Input: dimensioned drawing with shaded views. Units: mm. Origin: part minimum x, y, z. A direction names the side the tool comes from. Coordinates: 2 decimals unless noted, no trailing zeros. Loops run counter-clockwise (first coordinate to the right, second up) from the corner with the lowest first, then second, coordinate; pieces in that order, holes last. Notation, with made-up numbers: (-29.75, 77.5) - (-4.75, 77.5) arc R12 cw to (-4.75, 92.5) - close; hole circle Ø5 at (32, -16.5). An arc over 180 degrees is marked (long way). Put each result on its own line as item: value. Start each with the question number.
1) Contact query for flat-ended pins moving along their axis: pin 1 Ø1 at (x, z) = (4, 11) entering from +Y (1 decimal); pin 2 Ø3 at (x, z) = (2, 16) entering from +Y; pin 3 Ø3 at (y, z) = (11, 13.5) entering from -X. Output: stop coordinate, or through.
2) Reachability of the marked faces 4 and 5 from +Z, -Z, +X, -X, +Y, -Y: full face, straight path, thin tool, end or side. Return the list, or none.
3) Section A-A on y = 3.5. Output: boundary loops of the cut face in (x, z).
4) Section D-D on y = 16. Output: boundary loops of the cut face in (x, z).
5) Material intervals for line 1 along Y through (x, z) = (4.4, 4); line 2 along Z through (x, y) = (3.2, 12); line 3 along Z through (x, y) = (4.55, 20.5), sorted ascending. Write a range as from..to.
6) Section C-C on x = 3.8. Output: boundary loops of the cut face in (y, z), and give its area (3 significant figures).
7) Section B-B on z = 4. Output: boundary loops of the cut face in (x, y).
8) Draft query along Z for the marked faces 1, 2 and 3. Return one class per face: +Z half, -Z half, draft (parallel to the pull), parting line (faces both ways), or undercut.
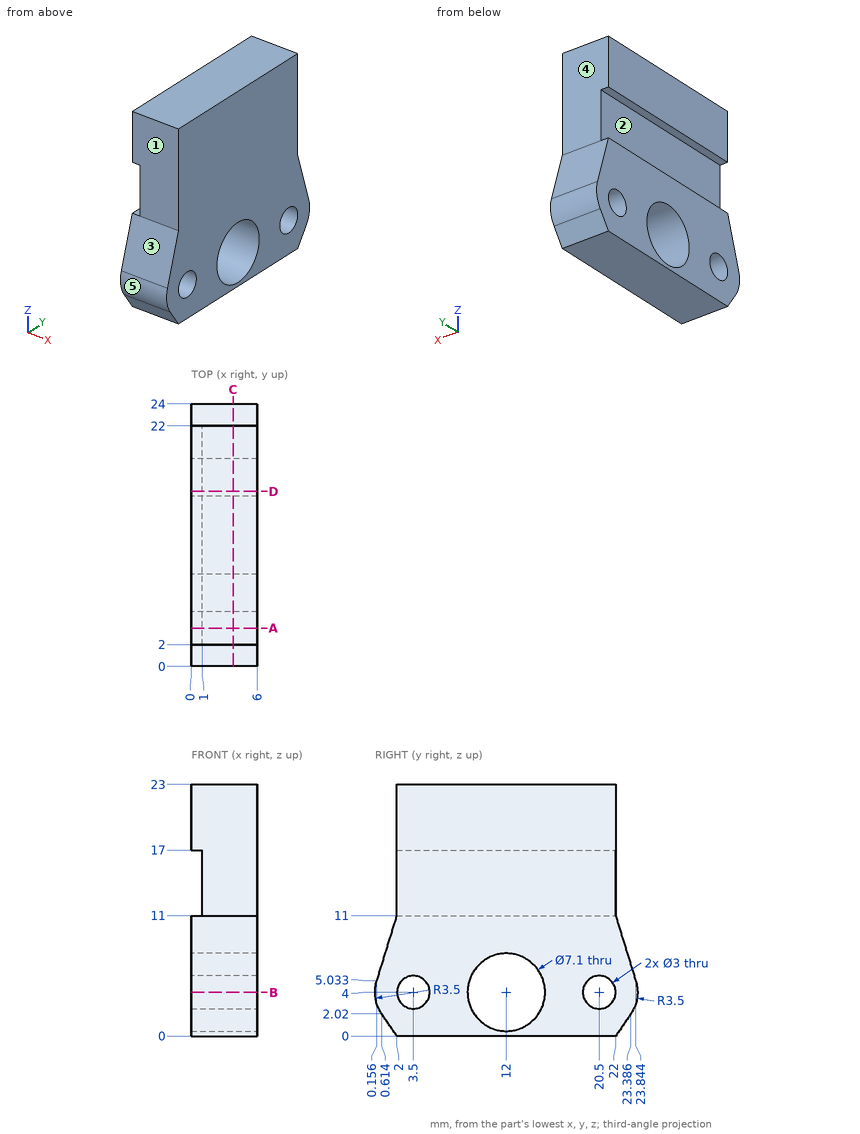
Answer block:
1. pin 1: stops at y = 22.2
1. pin 2: stops at y = 22
1. pin 3: stops at x = 1
2. face 4: +Z, +X, -X, +Y
2. face 5: +X, -X, -Y
3. outline: (0, 0) - (6, 0) - (6, 2.5) - (0, 2.5) - close; (0, 5.5) - (6, 5.5) - (6, 23) - (0, 23) - (0, 17) - (1, 17) - (1, 11) - (0, 11) - close
4. outline: (0, 0) - (6, 0) - (6, 23) - (0, 23) - (0, 17) - (1, 17) - (1, 11) - (0, 11) - close
5. line 1: y = 0..2, 5..8.45, 15.55..19, 22..24
5. line 2: z = 0..0.45, 7.55..23
5. line 3: z = 0..2.5, 5.5..23
6. outline: (0.16, 5.03) arc R3.5 ccw to (0.61, 2.02) - (2, 0) - (22, 0) - (23.39, 2.02) arc R3.5 ccw to (23.84, 5.03) - (22, 11) - (22, 23) - (2, 23) - (2, 11) - close; hole circle Ø3 at (3.5, 4); hole circle Ø7.1 at (12, 4); hole circle Ø3 at (20.5, 4)
6. area: 431 mm²
7. outline: (0, 0) - (6, 0) - (6, 2) - (0, 2) - close; (0, 5) - (6, 5) - (6, 8.45) - (0, 8.45) - close; (0, 15.55) - (6, 15.55) - (6, 19) - (0, 19) - close; (0, 22) - (6, 22) - (6, 24) - (0, 24) - close
8. face 1: draft
8. face 2: undercut
8. face 3: +Z half
